Source: CAD feature listing. Evaluate the final solid. Frame: model axes, mm. A direction names the side the tool comes from. Give positions to 0.01 mm unless a question says otherwise; leave off trailing zeros. Order: outer loops, then holes, each group sorted by start corner. A loop starts at its lowest first (then second) coordinate and runs counter-clockwise, first axis right, second up.
```python
from build123d import *

# Parameters (mm, degrees)
IZIM1_R                     = 5
IZIM1_R_2                   = 2.5
Y_KSEKLIK_EKSTR_ZYON2_DEPTH = 1
IZIM2_R                     = 3
Y_KSEKLIK_EKSTR_ZYON4_DEPTH = 1


with BuildPart() as part:
    # Çizim1 → Yükseklik-Ekstrüzyon2 (new body)
    with BuildSketch(Plane.XY):
        with BuildLine():
            Line((-25, 43.301270189), (-26.146521576, 40.39207739))
            ThreePointArc((-26.146521576, 40.39207739), (-27.544598222, 38.602623821), (-29.691484877, 37.862596744))
            Line((-29.691484877, 37.862596744), (-32.693673826, 37.730024144))
            Line((-32.693673826, 37.730024144), (-33.252115355, 34.777253066))
            ThreePointArc((-33.252115355, 34.777253066), (-34.290118058, 32.757522199), (-36.260310201, 31.628316593))
            Line((-36.260310201, 31.628316593), (-39.184480502, 30.935538106))
            Line((-39.184480502, 30.935538106), (-39.17973637, 27.930427214))
            ThreePointArc((-39.17973637, 27.930427214), (-39.820893366, 25.751969023), (-41.54459596, 24.273587558))
            Line((-41.54459596, 24.273587558), (-44.287157421, 23.045145208))
            Line((-44.287157421, 23.045145208), (-43.719395692, 20.094152054))
            ThreePointArc((-43.719395692, 20.094152054), (-43.940993675, 17.834139505), (-45.357143694, 16.058954583))
            Line((-45.357143694, 16.058954583), (-47.82093971, 14.338366552))
            Line((-47.82093971, 14.338366552), (-46.710273625, 11.546031539))
            ThreePointArc((-46.710273625, 11.546031539), (-46.504462376, 9.284526705), (-47.562892001, 7.275425136))
            Line((-47.562892001, 7.275425136), (-49.660641368, 5.123644113))
            Line((-49.660641368, 5.123644113), (-48.046416828, 2.588887101))
            ThreePointArc((-48.046416828, 2.588887101), (-47.420487313, 0.406004917), (-48.083701146, -1.765839874))
            Line((-48.083701146, -1.765839874), (-49.741090048, -4.272585973))
            Line((-49.741090048, -4.272585973), (-47.680491761, -6.459969953))
            ThreePointArc((-47.680491761, -6.459969953), (-46.656617846, -8.486899797), (-46.901121207, -10.744549126))
            Line((-46.901121207, -10.744549126), (-48.059435816, -13.517457571))
            Line((-48.059435816, -13.517457571), (-45.625461503, -15.279979352))
            ThreePointArc((-45.625461503, -15.279979352), (-44.239914432, -17.079151855), (-44.057045667, -19.342627369))
            Line((-44.057045667, -19.342627369), (-44.675252109, -22.283466496))
            Line((-44.675252109, -22.283466496), (-41.954126526, -23.558687864))
            ThreePointArc((-41.954126526, -23.558687864), (-40.255989993, -25.066366444), (-39.652227319, -27.255483394))
            Line((-39.652227319, -27.255483394), (-39.708425324, -30.260072511))
            Line((-39.708425324, -30.260072511), (-36.7965457, -31.002818113))
            ThreePointArc((-36.7965457, -31.002818113), (-34.84597704, -32.165592505), (-33.842709051, -34.202800331))
            Line((-33.842709051, -34.202800331), (-33.334907776, -37.164700371))
            Line((-33.334907776, -37.164700371), (-30.335428898, -37.348658075))
            ThreePointArc((-30.335428898, -37.348658075), (-28.201527977, -38.125336415), (-26.834295942, -39.938466016))
            Line((-26.834295942, -39.938466016), (-25.73775467, -42.866863479))
            ThreePointArc((-25.73775467, -42.866863479), (-24.554196145, -43.55561332), (-23.352220135, -44.21169319))
            ThreePointArc((-23.352220135, -44.21169319), (-17.219408632, -49.939828574), (-14.829333353, -57.984109281))
            ThreePointArc((-14.829333353, -57.984109281), (-20.099106379, -76.543069457), (-25, -57.883306535))
            Line((-25, -57.883306535), (-25, -57.052607302))
            ThreePointArc((-25, -57.052607302), (-25.590454576, -54.960957236), (-27.1875, -53.486819346))
            ThreePointArc((-27.1875, -53.486819346), (-59.999999835, 0.004450967), (-27.179564099, 53.490852446))
            ThreePointArc((-27.179564099, 53.490852446), (-24.232021318, 53.76021953), (-21.906244367, 51.929556087))
            ThreePointArc((-21.906244367, 51.929556087), (-21.212806241, 47.755648425), (-23.446136356, 44.161959762))
            ThreePointArc((-23.446136356, 44.161959762), (-24.226890609, 43.73851588), (-25, 43.301270189))
        make_face()
        with Locations((-20, -66.543560573)):
            Circle(IZIM1_R, mode=Mode.SUBTRACT)
        with Locations((-31.620079453, -45.001895242)):
            Circle(IZIM1_R_2, mode=Mode.SUBTRACT)
        with Locations((-55, 0)):
            Circle(IZIM1_R_2, mode=Mode.SUBTRACT)
        with Locations((-28.000624989, 47.338831842)):
            Circle(IZIM1_R_2, mode=Mode.SUBTRACT)
    extrude(amount=Y_KSEKLIK_EKSTR_ZYON2_DEPTH)

    # Çizim2 → Yükseklik-Ekstrüzyon4 (add)
    with BuildSketch(Plane.XY.offset(1)):
        with BuildLine():
            Line((-14.268162917, -55.859645389), (-13.746523784, -58.818007922))
            ThreePointArc((-13.746523784, -58.818007922), (-13.437306239, -59.381637082), (-12.848871774, -59.640554443))
            Line((-12.848871774, -59.640554443), (-9.856302857, -59.902370298))
            ThreePointArc((-9.856302857, -59.902370298), (-8.217998769, -61.049523171), (-8.392310254, -63.041912567))
            Line((-8.392310254, -63.041912567), (-10.115333894, -65.502645344))
            ThreePointArc((-10.115333894, -65.502645344), (-10.295230071, -66.119841167), (-10.062226293, -66.71900939))
            Line((-10.062226293, -66.71900939), (-8.131292285, -69.02020693))
            ThreePointArc((-8.131292285, -69.02020693), (-7.78399593, -70.989822436), (-9.316084816, -72.275397656))
            Line((-9.316084816, -72.275397656), (-12.274447349, -72.797036789))
            ThreePointArc((-12.274447349, -72.797036789), (-12.838076508, -73.106254334), (-13.09699387, -73.694688799))
            Line((-13.09699387, -73.694688799), (-13.358809725, -76.687257716))
            ThreePointArc((-13.358809725, -76.687257716), (-14.505962597, -78.325561805), (-16.498351994, -78.151250319))
            Line((-16.498351994, -78.151250319), (-18.95908477, -76.428226679))
            ThreePointArc((-18.95908477, -76.428226679), (-19.576280594, -76.248330502), (-20.175448817, -76.48133428))
            Line((-20.175448817, -76.48133428), (-22.476646357, -78.412268288))
            ThreePointArc((-22.476646357, -78.412268288), (-24.446261863, -78.759564643), (-25.731837083, -77.227475757))
            Line((-25.731837083, -77.227475757), (-26.253476216, -74.269113224))
            ThreePointArc((-26.253476216, -74.269113224), (-26.562693761, -73.705484065), (-27.151128226, -73.446566704))
            Line((-27.151128226, -73.446566704), (-30.143697143, -73.184750849))
            ThreePointArc((-30.143697143, -73.184750849), (-31.782001231, -72.037597976), (-31.607689746, -70.04520858))
            Line((-31.607689746, -70.04520858), (-29.884666106, -67.584475803))
            ThreePointArc((-29.884666106, -67.584475803), (-29.704769929, -66.967279979), (-29.937773707, -66.368111757))
            Line((-29.937773707, -66.368111757), (-31.868707715, -64.066914216))
            ThreePointArc((-31.868707715, -64.066914216), (-32.21600407, -62.09729871), (-30.683915184, -60.811723491))
            Line((-30.683915184, -60.811723491), (-27.725552651, -60.290084357))
            ThreePointArc((-27.725552651, -60.290084357), (-27.161923492, -59.980866812), (-26.90300613, -59.392432347))
            Line((-26.90300613, -59.392432347), (-26.641190275, -56.39986343))
            ThreePointArc((-26.641190275, -56.39986343), (-25.494037403, -54.761559342), (-23.501648006, -54.935870827))
            Line((-23.501648006, -54.935870827), (-21.04091523, -56.658894467))
            ThreePointArc((-21.04091523, -56.658894467), (-20.423719406, -56.838790644), (-19.824551183, -56.605786866))
            Line((-19.824551183, -56.605786866), (-17.523353643, -54.674852858))
            ThreePointArc((-17.523353643, -54.674852858), (-15.553738137, -54.327556503), (-14.268162917, -55.859645389))
        make_face()
        with Locations((-20, -66.543560573)):
            Circle(IZIM2_R, mode=Mode.SUBTRACT)
    extrude(amount=-Y_KSEKLIK_EKSTR_ZYON4_DEPTH)


solid = part.part
```
1) Material intervals for L1, parallel to Y at x = -49.5, z = 0.4; L2, parallel to Y at x = -35, z = 0.9; L3, parallel to Y at x = -20, z = 0.5, sorted ascending.
Report:
L1: y = -33.91 to -4.53, -3.91 to 4.87, 5.29 to 33.91
L2: y = -48.73 to -32.01, 32.17 to 48.73
L3: y = -76.54 to -69.54, -63.54 to -46.58
2) Section query C-C, the plane z = 0.35. Count the separate pieces of the cut face and the enclosed holes in it, and give its area (3 significant figures).
Report:
separate pieces: 1
enclosed holes: 4
area: 1,820 mm2
3) Section query B-B, the plane y = 0. Return the cut outline in (x, z).
Report:
outline: (-60, 0) - (-57.5, 0) - (-57.5, 1) - (-60, 1) - close; (-52.5, 0) - (-47.44, 0) - (-47.44, 1) - (-52.5, 1) - close
4) Pin query (flat end, axial travel): pin 1 (4 mm diameter, centred on x = -31.62, y = -45, fed in from -Z). Return the tip coordinate at first contact, or that it passes through.
Report:
pin 1: passes through
5) Section query A-A, the plane x = -55. Return the cut outline in (y, z), and give its area (3 significant figures).
Report:
outline: (-23.98, 0) - (-2.5, 0) - (-2.5, 1) - (-23.98, 1) - close; (2.5, 0) - (23.98, 0) - (23.98, 1) - (2.5, 1) - close
area: 43.0 mm2
6) Draft query along Y for faces 3 (the cylindrical face through (-27.52, 38.62, 0.49)), 4 (the flat face through (-45, -17, 0)). Return one class per face: +Y half, -Y half, draft (parallel to the pull), parting line (faces both ways), or undercut.
Report:
face 3: undercut
face 4: draft
7) Reachability of faces 1 (the cylindrical face through (-59.993, -0.92, 0.493)), 2 (the cylindrical face through (-34.87, -32.14, 0.49)) from +Z, -Z, +X, -X, +Y, -Y: full face, straight path, thin tool, end or side. Return the list, or none.
Report:
face 1: +Z, -Z, -X
face 2: +Z, -Z, +X
